Autodesk Inventor part; units mm, degrees
ref_plane "YZ Plane" through (0, 0, 0) normal (1, 0, 0) x (0, 1, 0)
ref_plane "XZ Plane" through (0, 0, 0) normal (0, 1, 0) x (-1, 0, 0)
ref_plane "XY Plane" through (0, 0, 0) normal (0, 0, 1) x (1, 0, 0)
sketch "Sketch1" plane through (0, 0, 0) normal (1, 0, 0) x (0, 1, 0)
  circle A0 centre (0, 0) radius 14.2875
  circle A1 centre (0, 0) radius 4.7625
  dimension "d0" = 28.575
  dimension "d2" = 9.525
extrude "Extrusion1" add sketch "Sketch1" along normal mid plane 12.7
sketch "Sketch2" plane through (6.35, 0, 0) normal (1, 0, 0) x (0, 0, -1)
  circle A0 centre (0, 0) radius 17.4625
  circle A1 centre (0, 0) radius 14.2875 construction
  circle A2 centre (0, 0) radius 4.7625
  dimension "d6" = 3.175
extrude "Extrusion2" add sketch "Sketch2" along normal blind 1.5875
sketch "Sketch3" plane through (-6.35, 0, 0) normal (-1, 0, 0) x (0, 0, 1)
  circle A0 centre (0, 0) radius 17.4625
  circle A1 centre (0, 0) radius 4.7625
extrude "Extrusion3" add sketch "Sketch3" along normal blind 1.5875
sketch "Sketch4" plane through (7.9375, 0, 0) normal (1, 0, 0) x (0, 0, -1)
  circle A0 centre (0, 0) radius 4.7625
  circle A1 centre (0, 0) radius 9.525
  dimension "d11" = 4.7625
extrude "Extrusion4" [suppressed]
properties part number "pulley XL 1.375in 2" material "Nylon 6/6"
Verification items for the finished model (mm, model axes). A direction names the side the tool comes from. Coordinates: 2 decimals unless noted, no trailing zeros. Order: outer loops, then holes, each group sorted by start corner. A loop starts at its lowest first (then second) coordinate and runs counter-clockwise, first axis right, second up. Notation, with made-up numbers: M 30,-9 L 76,-9 A14 cw 76,11 Z; hole C 64.25,79 d10. An arc over 180 degrees is marked long. Write each question's results on one line, items separated by ' | '.
1) Section check C-C on x = 4. Record the cut outline in (y, z) (1 decimal), plus the area to 3 significant figures.
Solved:
outline: C 0,0 d28.6; hole C 0,0 d9.5 | area: 570 mm²
2) Section check D-D on z = 10.5. Record the cut outline in (x, y).
Solved:
outline: M -7.94,-13.95 L -6.35,-13.95 L -6.35,-9.69 L 6.35,-9.69 L 6.35,-13.95 L 7.94,-13.95 L 7.94,13.95 L 6.35,13.95 L 6.35,9.69 L -6.35,9.69 L -6.35,13.95 L -7.94,13.95 Z
3) Access from +Z, -Z, +X, -X, +Y, -Y to the whole of each face (thin tool, end or side, straight path). Record for faces 1 (the face through (-6.35, -13, -7)), 2 (the face through (-7.938, -4, 4)).
Solved:
face 1: none | face 2: +Z, -Z, -X, +Y, -Y
4) Release check for a two-part mould opening along X. For faces 3 (the face through (7.938, -4, -4)), 4 (the face through (-7.133, 10.626, -13.858)), 5 (the face through (6.35, -13, 7)) record: pulls with the +X half, pulls with the -X half, needs draft (parallel to the pull), parting line crosses it, or undercut.
Solved:
face 3: pulls with the +X half | face 4: needs draft | face 5: undercut
5) Section check A-A on z = 0. Record the cut outline in (x, y).
Solved:
outline: M -7.94,-17.46 L -6.35,-17.46 L -6.35,-14.29 L 6.35,-14.29 L 6.35,-17.46 L 7.94,-17.46 L 7.94,-4.76 L -7.94,-4.76 Z; M -7.94,4.76 L 7.94,4.76 L 7.94,17.46 L 6.35,17.46 L 6.35,14.29 L -6.35,14.29 L -6.35,17.46 L -7.94,17.46 Z
6) Scan lines: line 1 along X through (y, z) = (-11, -12); line 2 along Z through (x, y) = (5.25, 0); line 3 along Y through (x, z) = (6.9, 0). Record each from-to range of solid material in increasing order. Write a range as [from, to].
Solved:
line 1: x = [-7.94, -6.35], [6.35, 7.94] | line 2: z = [-14.29, -4.76], [4.76, 14.29] | line 3: y = [-17.46, -4.76], [4.76, 17.46]
7) Gauge pin test, flat ends, axial feed: pin 1 Ø5.5 at (y, z) = (0, 0) entering from +X; pin 2 Ø2 at (x, y) = (5.5, -3.5) entering from -Z; pin 3 Ø2 at (x, z) = (0, 6.5) entering from -Y; pin 4 Ø1 at (x, z) = (-3, 10.5) entering from +Y. Record the tip position at first contact, or that the pin passes through.
Solved:
pin 1: passes through | pin 2: stops at z = -17.21 | pin 3: stops at y = -13.19 | pin 4: stops at y = 10.2
